Source: three-view drawing plus pictorial views. Frame: mm from the lowest corner of the part. Round coordinates to 2 decimals unless told otherwise and drop trailing zeros. Order: outer loops, then holes, each group sorted by start corner. A loop starts at its lowest first (then second) coordinate and runs counter-clockwise, first axis right, second up. Notation, with made-up numbers: (80, 40.25) -> (94, 40.25) arc R31 cw to (94, 76.25) -> close; hole circle Ø1 at (-1.75, -11). An arc over 180 degrees is marked (long way). Use a Markdown table: item, result.
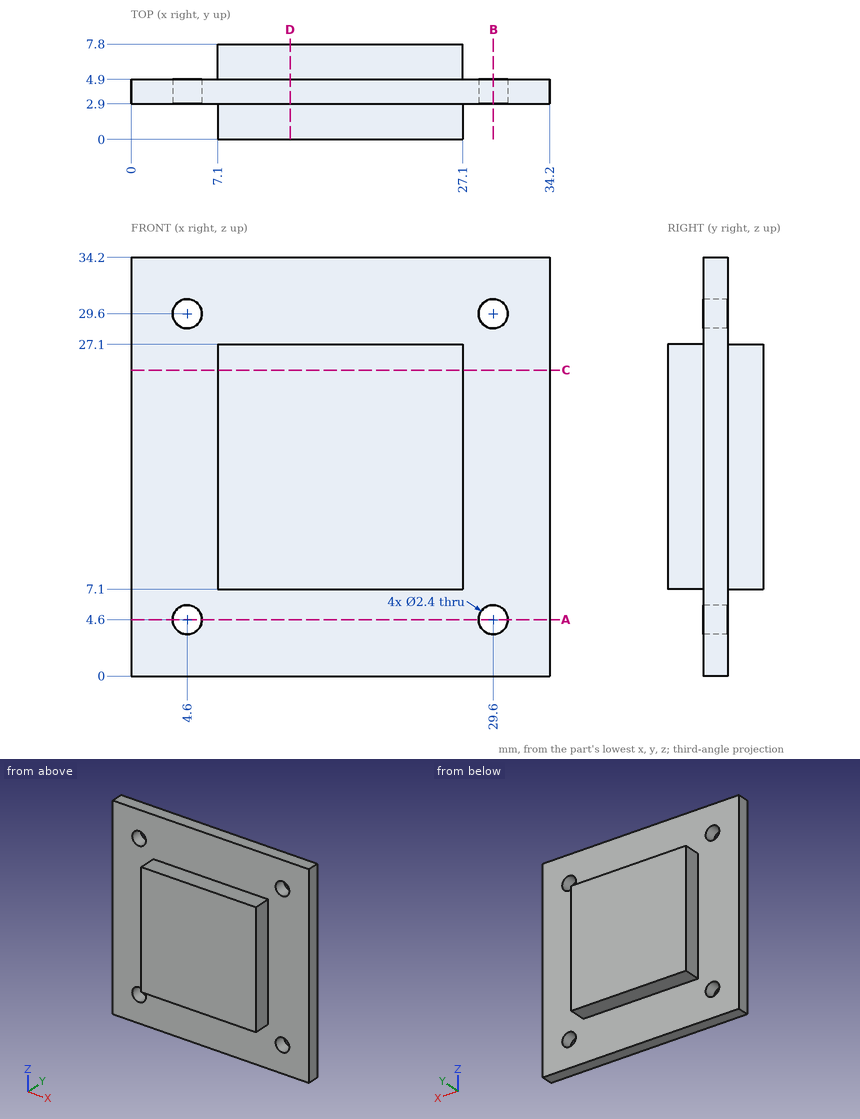
1) Cut plane A-A on z = 4.6. Return loops of the section in (x, y).
Results found:
| item | result |
|---|---|
| outline | (0, 2.9) -> (3.4, 2.9) -> (3.4, 4.9) -> (0, 4.9) -> close; (5.8, 2.9) -> (28.4, 2.9) -> (28.4, 4.9) -> (5.8, 4.9) -> close; (30.8, 2.9) -> (34.2, 2.9) -> (34.2, 4.9) -> (30.8, 4.9) -> close |
2) Cut plane C-C on z = 25. Return loops of the section in (x, y), and give its area (3 significant figures).
Results found:
| item | result |
|---|---|
| outline | (0, 2.9) -> (7.1, 2.9) -> (7.1, 0) -> (27.1, 0) -> (27.1, 2.9) -> (34.2, 2.9) -> (34.2, 4.9) -> (27.1, 4.9) -> (27.1, 7.8) -> (7.1, 7.8) -> (7.1, 4.9) -> (0, 4.9) -> close |
| area | 184 mm² |
3) Pin query (flat end, axial travel): pin 1 Ø1.4 at (y, z) = (1, 16) entering from +X; pin 2 Ø3 at (x, y) = (13.5, 2) entering from +Z; pin 3 Ø0.9 at (x, y) = (17, 7) entering from -Z; pin 4 Ø3 at (y, z) = (1, 4.5) entering from -X. Return the tip coordinate at first contact, or that it passes through.
Results found:
| item | result |
|---|---|
| pin 1 | stops at x = 27.1 |
| pin 2 | stops at z = 34.2 |
| pin 3 | stops at z = 7.1 |
| pin 4 | passes through |
4) Cut plane B-B on x = 29.6. Return loops of the section in (y, z).
Results found:
| item | result |
|---|---|
| outline | (2.9, 0) -> (4.9, 0) -> (4.9, 3.4) -> (2.9, 3.4) -> close; (2.9, 5.8) -> (4.9, 5.8) -> (4.9, 28.4) -> (2.9, 28.4) -> close; (2.9, 30.8) -> (4.9, 30.8) -> (4.9, 34.2) -> (2.9, 34.2) -> close |
5) Line query: L1, parallel to Z at x = 29.6, y = 3.8; L2, parallel to X at y = 5.5, z = 12. Output: solid intervals per line, ascending. Write a range as [from, to].
Results found:
| item | result |
|---|---|
| L1 | z = [0, 3.4], [5.8, 28.4], [30.8, 34.2] |
| L2 | x = [7.1, 27.1] |
6) Cut plane D-D on x = 13. Return loops of the section in (y, z).
Results found:
| item | result |
|---|---|
| outline | (0, 7.1) -> (2.9, 7.1) -> (2.9, 0) -> (4.9, 0) -> (4.9, 7.1) -> (7.8, 7.1) -> (7.8, 27.1) -> (4.9, 27.1) -> (4.9, 34.2) -> (2.9, 34.2) -> (2.9, 27.1) -> (0, 27.1) -> close |
